Can you work these out from the model? Positions are in its coordinate system, mm. A direction names the side the tool comes from. Give positions to 0.01 mm unless a question says otherwise; leave off trailing zeros. Loops run counter-clockwise (first coordinate to the right, second up) from the corner with the lowest first, then second, coordinate; pieces in that order, holes last. Notation, with made-up numbers: M 37,82.25 L 92,82.25 A14 cw 92,102.25 Z; hole C 24,42.25 d5. An arc over 180 degrees is marked long. Put each result on its own line as item: value. Start each with the question number.
1) For faces 1 (the cylindrical face through (36.83, 10.6, -7.28)), 2 (the flat face through (3, 3, -2)), 3 (the flat face through (3, 5, -7)), 4 (the flat face through (3, 3, -11)), which set-ups out of +Z, -Z, +X, -X, +Y, -Y let a thin tool reach every point of the face, with its end or its side?
2) Imagine slicing it at D-D (x = 57). Write out the boundary of the cut face in (y, z).
3) For P1, Ø6.5, axis at x = 55.5, z = -9.5, coming from the +Y side; P2, Ø1, axis at x = 4, y = 4, coming from the -Z side; P3, Ø1.7, axis at y = 3, z = -6, coming from the +X side, each with a flat end and sliding along its axis, tell me the tip position at first contact or that it passes through.
4) If we mould it in two halves opening along Z, with no side actions, what happens to faces 5 (the flat face through (15, 1.6, -7)), 6 (the cylindrical face through (12.054, 0.789, -1.328)), 7 (the flat face through (31, 2, 0)), 8 (the cylindrical face through (11.845, 0.789, -11.921))? For each: +Z half, -Z half, draft (parallel to the pull), parting line (faces both ways), or undercut.
5) Imagine slicing it at B-B (x = 11). Write out the boundary of the cut face in (y, z), then the cut area to 3 significant figures.
6) Imagine slicing it at A-A (y = 3.25). Write out the boundary of the cut face in (x, z), then the cut area to 3 significant figures.
7) Imagine slicing it at C-C (z = -6.5). Write out the boundary of the cut face in (x, y), then the cut area to 3 significant figures.
8) Please list where these lines run through material, in increasing order: line 1 along X through (y, z) = (0.6, -11); line 2 along X through (y, z) = (4.5, -6); line 3 along X through (y, z) = (6.75, -4). Write a range as from..to.
from build123d import *

# Parameters (mm, degrees)
SKETCH1_W             = 24.62
SKETCH1_H             = 13
SKETCH1_R             = 1.25
BOSS_EXTRUDE1_DEPTH   = 1.6
SKETCH1_W_2           = 24.38
BOSS_EXTRUDE1_2_DEPTH = 1.6
SKETCH1_3_W           = 13
SKETCH1_3_H           = 13
BOSS_EXTRUDE2_DEPTH   = 6.9
SKETCH1_4_R           = 6
BOSS_EXTRUDE3_DEPTH   = 14.4
SKETCH3_W             = 7
SKETCH3_H             = 9
BOSS_EXTRUDE4_DEPTH   = 3.4


with BuildPart() as part:
    # Sketch1 → Boss-Extrude1 (new body)
    with BuildSketch(Plane(origin=(0, 0, 0), x_dir=(1, 0, 0), z_dir=(0, 1, 0))):
        with Locations((49.69, 6.5)):
            Rectangle(SKETCH1_W, SKETCH1_H)
        with Locations(Location((60, 2, 0), (0, 0, 270))):
            Circle(SKETCH1_R, mode=Mode.SUBTRACT)
        with Locations(Location((60, 11, 0), (0, 0, 270))):
            Circle(SKETCH1_R, mode=Mode.SUBTRACT)
    extrude(amount=BOSS_EXTRUDE1_DEPTH)



with BuildPart() as body_2:
    # Sketch1 → Boss-Extrude1 2 (new body)
    with BuildSketch(Plane(origin=(0, 0, 0), x_dir=(1, 0, 0), z_dir=(0, 1, 0))):
        with Locations((12.19, 6.5)):
            Rectangle(SKETCH1_W_2, SKETCH1_H)
        with Locations(Location((11, 2, 0), (0, 0, 270))):
            Circle(SKETCH1_R, mode=Mode.SUBTRACT)
        with Locations(Location((11, 11, 0), (0, 0, 270))):
            Circle(SKETCH1_R, mode=Mode.SUBTRACT)
    extrude(amount=BOSS_EXTRUDE1_2_DEPTH)


with BuildPart() as part_1:
    add(part.part)

    add(body_2.part)  # Boss-Extrude2 merges body 2
    # Sketch1_3 → Boss-Extrude2 (add)
    with BuildSketch(Plane(origin=(0, 0, 0), x_dir=(1, 0, 0), z_dir=(0, 1, 0))):
        with Locations((30.88, 6.5)):
            Rectangle(SKETCH1_3_W, SKETCH1_3_H)
    extrude(amount=BOSS_EXTRUDE2_DEPTH)

    # Sketch1_4 → Boss-Extrude3 (add)
    with BuildSketch(Plane(origin=(0, 0, 0), x_dir=(1, 0, 0), z_dir=(0, 1, 0))):
        with Locations(Location((30.88, 6.5, 0), (0, 0, 270))):
            Circle(SKETCH1_4_R)
    extrude(amount=BOSS_EXTRUDE3_DEPTH)

    # Sketch3 → Boss-Extrude4 (add)
    with BuildSketch(Plane(origin=(0, 1.6, 0), x_dir=(1, 0, 0), z_dir=(0, 1, 0))):
        with Locations((3.5, 6.5)):
            Rectangle(SKETCH3_W, SKETCH3_H)
    extrude(amount=BOSS_EXTRUDE4_DEPTH)


solid = part_1.part
Recorded:
1. face 1: +Y
1. face 2: +Z, -X, +Y
1. face 3: +Z, -Z, -X, +Y
1. face 4: -Z, -X, +Y
2. outline: M 0,-13 L 1.6,-13 L 1.6,0 L 0,0 Z
3. P1: y = 1.6
3. P2: z = -11
3. P3: x = 37.38
4. face 5: draft
4. face 6: undercut
4. face 7: +Z half
4. face 8: undercut
5. outline: M 0,-13 L 1.6,-13 L 1.6,-12.25 L 0,-12.25 Z; M 0,-9.75 L 1.6,-9.75 L 1.6,-3.25 L 0,-3.25 Z; M 0,-0.75 L 1.6,-0.75 L 1.6,0 L 0,0 Z
5. area: 12.8 mm²
6. outline: M 0,-11 L 7,-11 L 7,-2 L 0,-2 Z; M 24.38,-13 L 37.38,-13 L 37.38,0 L 24.38,0 Z
6. area: 232 mm²
7. outline: M 0,0 L 62,0 L 62,1.6 L 37.38,1.6 L 37.38,6.9 L 36.88,6.9 L 36.88,14.4 L 24.88,14.4 L 24.88,6.9 L 24.38,6.9 L 24.38,1.6 L 7,1.6 L 7,5 L 0,5 Z
7. area: 282 mm²
8. line 1: 0..9.75, 12.25..58.75, 61.25..62
8. line 2: 0..7, 24.38..37.38
8. line 3: 24.38..37.38
